Geometry: final body of the model. Coordinates: model frame, mm. Round coordinates to 2 decimals unless told otherwise and drop trailing zeros. Loops run counter-clockwise (first coordinate to the right, second up) from the corner with the lowest first, then second, coordinate; pieces in that order, holes last. Notation, with made-up numbers: M 60,54 L 93,54 A29 ccw 93,92 Z; hole C -27.5,53 d9. An arc over 180 degrees is marked long. Answer as a JSON object with one key per item and string values.
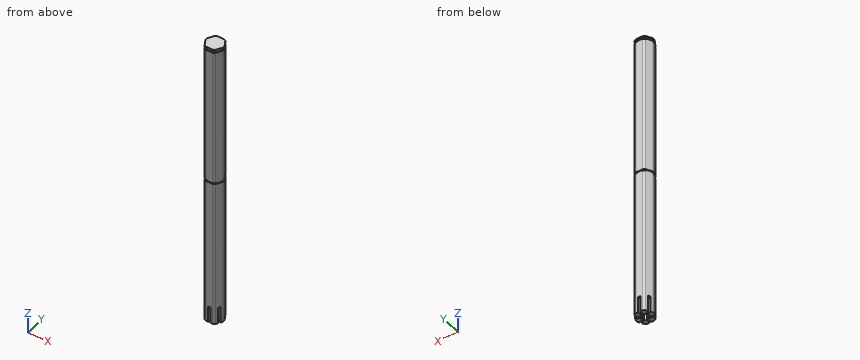
```python
from build123d import *

# Parameters (mm, degrees)
SKETCH2_OUTSIDE_W   = 40.204
SKETCH2_OUTSIDE_H   = 40.204
CUT_EXTRUDE1_DEPTH  = 114.289694924
BOSS_EXTRUDE1_START = 114.3
SKETCH3_R           = 2.4892
BOSS_EXTRUDE1_DEPTH = 114.3
SKETCH4_R           = 3.175
CUT_EXTRUDE2_DEPTH  = 12.7
SKETCH5_W           = 1.5748
SKETCH5_H           = 12.7
CUT_EXTRUDE3_DEPTH  = 12.7
CIRPATTERN1_COUNT   = 6


with BuildPart() as part:
    # Sketch1 → Revolve3 (revolve)
    with BuildSketch(Plane(origin=(0, 0, 0), x_dir=(0, 0, -1), z_dir=(1, 0, 0)), mode=Mode.PRIVATE) as revolve3_sk:
        Polygon((111.252, 7.62), (112.776, 7.62), (112.776, 0), (0, 0), (0, 7.62), (1.524, 7.62), (1.524, 5.9436), (2.5146, 5.9436), (2.5146, 7.62), (110.2614, 7.62), (110.2614, 5.9436), (111.252, 5.9436), align=None)
    revolve(revolve3_sk.sketch.rotate(Axis((0, 0, 0), (0, 0, -1)), 90), axis=Axis((0, 0, 0), (0, 0, -1)))

    # Sketch2 outside → Cut-Extrude1 (cut, through all)
    with BuildSketch(Plane(origin=(0, 0, -112.776), x_dir=(-1, 0, 0), z_dir=(0, 0, -1))):
        Rectangle(SKETCH2_OUTSIDE_W, SKETCH2_OUTSIDE_H)
        with BuildLine():
            Line((6.811131972, 0.902773368), (4.187390656, 5.447226632))
            ThreePointArc((4.187390656, 5.447226632), (3.43535, 5.950200742), (2.623741315, 6.35))
            Line((2.623741315, 6.35), (-2.623741315, 6.35))
            ThreePointArc((-2.623741315, 6.35), (-3.43535, 5.950200742), (-4.187390656, 5.447226632))
            Line((-4.187390656, 5.447226632), (-6.811131972, 0.902773368))
            ThreePointArc((-6.811131972, 0.902773368), (-6.8707, 0), (-6.811131972, -0.902773368))
            Line((-6.811131972, -0.902773368), (-4.187390656, -5.447226632))
            ThreePointArc((-4.187390656, -5.447226632), (-3.43535, -5.950200742), (-2.623741315, -6.35))
            Line((-2.623741315, -6.35), (2.623741315, -6.35))
            ThreePointArc((2.623741315, -6.35), (3.43535, -5.950200742), (4.187390656, -5.447226632))
            Line((4.187390656, -5.447226632), (6.811131972, -0.902773368))
            ThreePointArc((6.811131972, -0.902773368), (6.8707, 0), (6.811131972, 0.902773368))
        make_face(mode=Mode.SUBTRACT)
    extrude(amount=-CUT_EXTRUDE1_DEPTH, mode=Mode.SUBTRACT)

    # Sketch3 → Boss-Extrude1 (add)
    with BuildSketch(Plane(origin=(0, 0, -112.776), x_dir=(-1, 0, 0), z_dir=(0, 0, -1)).offset(BOSS_EXTRUDE1_START)):
        with BuildLine():
            Line((4.187390656, -5.447226632), (6.811131972, -0.902773368))
            ThreePointArc((6.811131972, -0.902773368), (6.8707, 0), (6.811131972, 0.902773368))
            Line((6.811131972, 0.902773368), (4.187390656, 5.447226632))
            ThreePointArc((4.187390656, 5.447226632), (3.43535, 5.950200742), (2.623741315, 6.35))
            Line((2.623741315, 6.35), (-2.623741315, 6.35))
            ThreePointArc((-2.623741315, 6.35), (-3.43535, 5.950200742), (-4.187390656, 5.447226632))
            Line((-4.187390656, 5.447226632), (-6.811131972, 0.902773368))
            ThreePointArc((-6.811131972, 0.902773368), (-6.8707, 0), (-6.811131972, -0.902773368))
            Line((-6.811131972, -0.902773368), (-4.187390656, -5.447226632))
            ThreePointArc((-4.187390656, -5.447226632), (-3.43535, -5.950200742), (-2.623741315, -6.35))
            Line((-2.623741315, -6.35), (2.623741315, -6.35))
            ThreePointArc((2.623741315, -6.35), (3.43535, -5.950200742), (4.187390656, -5.447226632))
        make_face()
        Circle(SKETCH3_R, mode=Mode.SUBTRACT)
    extrude(amount=-BOSS_EXTRUDE1_DEPTH)

    # Sketch4 → Cut-Extrude2 (cut)
    with BuildSketch(Plane(origin=(0, 0, -227.076), x_dir=(-1, 0, 0), z_dir=(0, 0, -1))):
        Circle(SKETCH4_R)
    extrude(amount=-CUT_EXTRUDE2_DEPTH, mode=Mode.SUBTRACT)

    # Sketch5 → Cut-Extrude3 (cut)
    with BuildSketch(Plane(origin=(0, 0, -227.076), x_dir=(-1, 0, 0), z_dir=(0, 0, -1))):
        Rectangle(SKETCH5_W, SKETCH5_H)
    cut_extrude3 = extrude(amount=-CUT_EXTRUDE3_DEPTH, mode=Mode.SUBTRACT)

    # CirPattern1: Cut-Extrude3 ×6 about axis
    cirpattern1_axis = Axis((0, 0, 0), (0, 0, 1))
    for i in range(1, CIRPATTERN1_COUNT):
        add(cut_extrude3.rotate(cirpattern1_axis, i * 360 / CIRPATTERN1_COUNT), mode=Mode.SUBTRACT)


solid = part.part
```
1) Line query: probe 1 along Z at (x, y) = (3.5, 5); probe 2 along X at (y, z) = (0, -142.5); probe 3 along Y at (x, z) = (-0.25, -160). Output: solid intervals per line, ascending.
Geometry results:
{"probe 1": "-227.08 to -111.25, -110.26 to -2.51, -1.52 to 0", "probe 2": "-6.87 to -2.49, 2.49 to 6.87", "probe 3": "-6.35 to -2.48, 2.48 to 6.35"}
2) First-contact query: pin 1 (2.5 mm diameter, centred on y = -5.5, z = -221.5, fed in from +X); pin 2 (1 mm diameter, centred on y = 4, z = -157.5, fed in from +X); pin 3 (1 mm diameter, centred on y = 4.5, z = -221, fed in from -X). Flat tips, straight axial feed; report the tip coordinate or a pass-through.
Geometry results:
{"pin 1": "x = 4.88", "pin 2": "x = 5.31", "pin 3": "x = -5.02"}
3) Cut plane A-A on z = -197. Return the cut outline in (x, y).
Geometry results:
{"outline": "M -6.81,-0.9 L -4.19,-5.45 A6.87 ccw -2.62,-6.35 L 2.62,-6.35 A6.87 ccw 4.19,-5.45 L 6.81,-0.9 A6.87 ccw 6.81,0.9 L 4.19,5.45 A6.87 ccw 2.62,6.35 L -2.62,6.35 A6.87 ccw -4.19,5.45 L -6.81,0.9 A6.87 ccw Z; hole C 0,0 d4.98"}
